Geometry: final body of the model. Coordinates: model frame, mm. A direction names the side the tool comes from. Give positions to 0.01 mm unless a question says otherwise; leave off trailing zeros. Order: outer loops, then holes, each group sorted by start corner. A loop starts at its lowest first (then second) coordinate and runs counter-clockwise, first axis right, second up. Notation, with made-up numbers: (-36.5, 35) -> (-7.5, 35) arc R22 cw to (-7.5, 57) -> close; hole circle Ø5 at (-3.5, 50). An arc over 180 degrees is marked (long way). Answer in a Markdown table with one row per item. Add a question column.
Q1. Set-up query: faces 5 (the face through (0, 0, -7)), 6 (the face through (0, -46, -8)), 7 (the face through (10, -23, -20)), 8 (the face through (-7.5, -23, -19)), 9 (the face through (0, -48, -17)). Return all of +Z, -Z, +X, -X, +Y, -Y with unobstructed straight access to the full face (end or side cutting, diameter ignored); none if empty.
Q2. Pull-direction query (X, two-part tool) for faces 1 (the face through (-13, -23, -10)), 2 (the face through (0, 2, -17)), 3 (the face through (13, -23, -10)), 4 (the face through (0, -23, -18)); classes: +X half, -X half, draft (parallel to the pull), parting line (faces both ways), or undercut.
Q3. Line query: line 1 along Y through (x, z) = (5.25, -11.75); line 2 along Z through (x, y) = (-5, -16). Output: solid intervals per line, ascending. Write a range as from..to.
Q4. Cut plane B-B on y = -2.5. Return the cut outline in (x, z).
Q5. Cut plane C-C on z = -4.75. Return the cut outline in (x, y).
Q6. Contact query for flat-ended pins moving along their axis: P1, Ø1.6, axis at x = -5.5, y = 1, coming from the +Z side; P2, Ø1, axis at x = 8.5, z = -13.5, coming from the +Y side; P3, Ø12, axis at x = 1.5, z = -4.5, coming from the -Y side. Output: stop coordinate, or through.
Q7. Cut plane A-A on x = -9. Return the cut outline in (y, z), and give its area (3 significant figures).
from build123d import *

# Parameters (mm, degrees)
EXTRUDE_1_DEPTH     = 13
SKETCH_4_W          = 20
SKETCH_4_H          = 60
CUT_EXTRUDE_1_DEPTH = 7.5


with BuildPart() as part:
    # 스케치2 → 보스-돌출1 (new, symmetric)
    with BuildSketch(Plane(origin=(0, 0, 0), x_dir=(0, 0, -1), z_dir=(1, 0, 0))):
        Polygon((0, 0), (15, 0), (15, 2), (20, 2), (20, -48), (15, -48), (15, -46), (0, -46), align=None)
    extrude(amount=EXTRUDE_1_DEPTH, both=True)

    # 스케치4 → 컷-돌출1 (cut, symmetric)
    with BuildSketch(Plane(origin=(0, 0, 0), x_dir=(0, 0, -1), z_dir=(1, 0, 0))):
        with Locations((28, -23.786029553)):
            Rectangle(SKETCH_4_W, SKETCH_4_H)
    extrude(amount=CUT_EXTRUDE_1_DEPTH, both=True, mode=Mode.SUBTRACT)


solid = part.part
Completed:
| question | item | result |
|---|---|---|
| 1 | face 5 | +Z, +X, -X, +Y |
| 1 | face 6 | +Z, +X, -X, -Y |
| 1 | face 7 | -Z, +X, -X, +Y, -Y |
| 1 | face 8 | -Z, +Y, -Y |
| 1 | face 9 | +Z, -Z, +X, -X, -Y |
| 2 | face 1 | -X half |
| 2 | face 2 | draft |
| 2 | face 3 | +X half |
| 2 | face 4 | undercut |
| 3 | line 1 | y = -46..0 |
| 3 | line 2 | z = -18..0 |
| 4 | outline | (-13, -20) -> (-7.5, -20) -> (-7.5, -18) -> (7.5, -18) -> (7.5, -20) -> (13, -20) -> (13, 0) -> (-13, 0) -> close |
| 5 | outline | (-13, -46) -> (13, -46) -> (13, 0) -> (-13, 0) -> close |
| 6 | P1 | stops at z = -15 |
| 6 | P2 | stops at y = 0 |
| 6 | P3 | stops at y = -46 |
| 7 | outline | (-48, -20) -> (2, -20) -> (2, -15) -> (0, -15) -> (0, 0) -> (-46, 0) -> (-46, -15) -> (-48, -15) -> close |
| 7 | area | 940 mm² |
